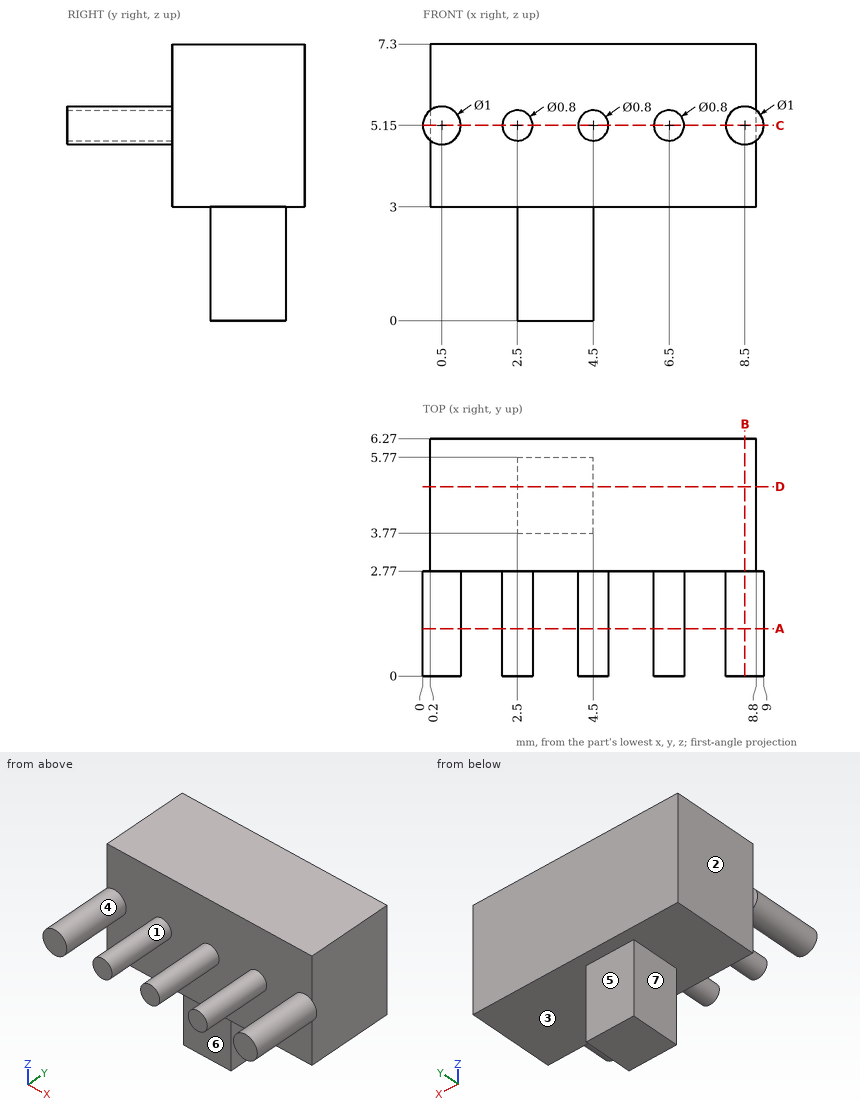
For this review, use the dimensioned drawing (mm, ordinates from the lowest corner) and the shaded views. A direction names the side the tool comes from. Coordinates: 2 decimals unless noted, no trailing zeros. Loops run counter-clockwise (first coordinate to the right, second up) from the corner with the lowest first, then second, coordinate; pieces in that order, holes last.
1. Add section C-C, the plane z = 5.15. Give the boundary of the cut face in (x, y), then the cut area to 3 significant figures.
2. Add section A-A, the plane y = 1.25. Give the boundary of the cut face in (x, z).
3. Add section B-B, the plane x = 8.5. Give the boundary of the cut face in (y, z), then the cut area to 3 significant figures.
4. Add section D-D, the plane y = 5. Give the boundary of the cut face in (x, z).
5. For line 1 (X direction, y = 0.5, z = 5.25); line 2 (X direction, y = 3.5, z = 3.25); line 3 (Y direction, x = 3.75, z = 0.5), list the stretches that pass through material, from the lowest coordinate up.
6. For the marked faces 4, 5, 6 and 7, list the 3-axis set-ups (+Z, -Z, +X, -X, +Y, -Y) from which the entire face can be reached by the end or side of a thin tool; tool diameter is ignored.
7. Mouldability with a two-part tool opening along X and no side actions: class the marked faces 1, 2 and 3 as +X half, -X half, draft (parallel to the pull), parting line (faces both ways), or undercut.
8. Insertion check: P1, Ø2, axis at x = 3, z = 1, coming from the -Y side; P2, Ø2, axis at x = 7, y = 4, coming from the -Z side; P3, Ø3, axis at y = 4.5, z = 5, coming from the -X side. Each pin has a flat end and moves straight along its axis. Give the tip position at first contact, or say it passes through.
Result:
1. outline: (0, 0) - (1, 0) - (1, 2.77) - (2.1, 2.77) - (2.1, 0) - (2.9, 0) - (2.9, 2.77) - (4.1, 2.77) - (4.1, 0) - (4.9, 0) - (4.9, 2.77) - (6.1, 2.77) - (6.1, 0) - (6.9, 0) - (6.9, 2.77) - (8, 2.77) - (8, 0) - (9, 0) - (9, 2.77) - (8.8, 2.77) - (8.8, 6.27) - (0.2, 6.27) - (0.2, 2.77) - (0, 2.77) - close
1. area: 42.3 mm2
2. outline: circle Ø1 at (0.5, 5.15); circle Ø0.8 at (2.5, 5.15); circle Ø0.8 at (4.5, 5.15); circle Ø0.8 at (6.5, 5.15); circle Ø1 at (8.5, 5.15)
3. outline: (0, 4.65) - (2.77, 4.65) - (2.77, 3) - (6.27, 3) - (6.27, 7.3) - (2.77, 7.3) - (2.77, 5.65) - (0, 5.65) - close
3. area: 17.8 mm2
4. outline: (0.2, 3) - (2.5, 3) - (2.5, 0) - (4.5, 0) - (4.5, 3) - (8.8, 3) - (8.8, 7.3) - (0.2, 7.3) - close
5. line 1: x = 0.01 to 0.99, 2.11 to 2.89, 4.11 to 4.89, 6.11 to 6.89, 8.01 to 8.99
5. line 2: x = 0.2 to 8.8
5. line 3: y = 3.77 to 5.77
6. face 4: -Y
6. face 5: -Z, +X, -X, +Y
6. face 6: -Z, +X, -X, -Y
6. face 7: -Z, -X, +Y, -Y
7. face 1: undercut
7. face 2: -X half
7. face 3: draft
8. P1: stops at y = 3.77
8. P2: stops at z = 3
8. P3: stops at x = 0.2
